```python
from build123d import *

# Parameters (mm, degrees)
ESQUISSE2_R        = 10
ESQUISSE2_R_2      = 1
BOSS_EXTRU_1_DEPTH = 2
BOSS_EXTRU_2_DEPTH = 2


with BuildPart() as part:
    # Esquisse2 → Boss.-Extru.1 (new body)
    with BuildSketch(Plane.XY):
        with Locations((22.149661623, 17.880169066)):
            Circle(ESQUISSE2_R)
        with Locations((16.492807374, 23.537023315)):
            Circle(ESQUISSE2_R_2, mode=Mode.SUBTRACT)
        with Locations((22.149661623, 25.880169066)):
            Circle(ESQUISSE2_R_2, mode=Mode.SUBTRACT)
        with Locations((27.806515873, 23.537023315)):
            Circle(ESQUISSE2_R_2, mode=Mode.SUBTRACT)
        with Locations((30.149661623, 17.880169066)):
            Circle(ESQUISSE2_R_2, mode=Mode.SUBTRACT)
        with Locations((27.806515873, 12.223314816)):
            Circle(ESQUISSE2_R_2, mode=Mode.SUBTRACT)
        with Locations((22.149661623, 9.880169066)):
            Circle(ESQUISSE2_R_2, mode=Mode.SUBTRACT)
        with Locations((16.492807374, 12.223314816)):
            Circle(ESQUISSE2_R_2, mode=Mode.SUBTRACT)
        with Locations((14.149661623, 17.880169066)):
            Circle(ESQUISSE2_R_2, mode=Mode.SUBTRACT)
    extrude(amount=BOSS_EXTRU_1_DEPTH)

    # Esquisse3 → Boss.-Extru.2 (add)
    with BuildSketch(Plane.XY.offset(2)):
        with BuildLine():
            ThreePointArc((26.149661623, 17.880169066), (24.978088748, 20.70859619), (22.149661623, 21.880169066))
            Line((22.149661623, 21.880169066), (22.149661623, 13.880169066))
            ThreePointArc((22.149661623, 13.880169066), (24.978088748, 15.051741941), (26.149661623, 17.880169066))
        make_face()
        with BuildLine():
            Line((22.149661623, 13.880169066), (22.149661623, 21.880169066))
            ThreePointArc((22.149661623, 21.880169066), (18.149661623, 17.880169066), (22.149661623, 13.880169066))
        make_face()
    extrude(amount=BOSS_EXTRU_2_DEPTH)


solid = part.part
```
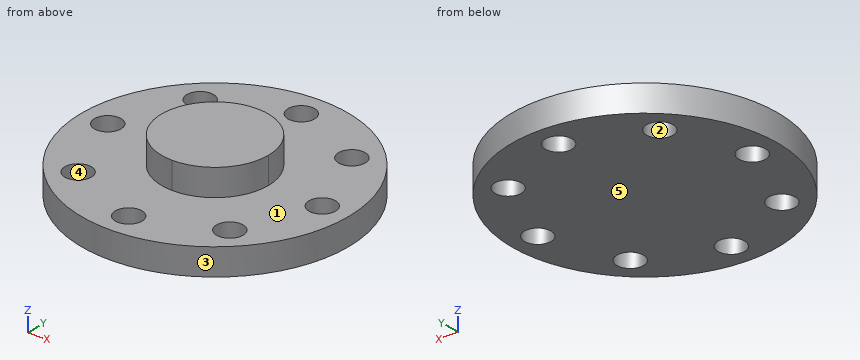
Design review of the part built by this model. Coordinates are the model's own, in mm. Face numbers are marked on the shaded views. A direction names the side the tool comes from. Coordinates: 2 decimals unless noted, no trailing zeros. Write each loop counter-clockwise with the first axis right and the second up, starting at its lowest first coordinate (ties: lowest second). Pieces come first, ordered by that corner, then holes.
1) Mouldability with a two-part tool opening along Y and no side actions: class the marked faces 3, 4 and 5 as +Y half, -Y half, draft (parallel to the pull), parting line (faces both ways), or undercut.
2) Machinability: for the marked faces 1 and 2, which of the approach directions +Z, -Z, +X, -X, +Y, -Y give a long, thin tool a straight path to every point of the face, cutting with its end or side? Answer none if there is none.
3) To check wall thickness, follow L1, parallel to Y at x = 22.5, z = 1.25; L2, parallel to Z at x = 21.25, y = 12.75; L3, parallel to X at y = 22.25, z = 0.2. State the ranges of each line that lie inside material, in increasing order.
4) Add section B-B (x = 30). Write out the cut boundary in (y, z), plus the area to 3 significant figures.
5) Add section D-D (x = 16). Write out the cut boundary in (y, z), plus the area to 3 significant figures.
6) Insertion check: pin 1 (2.5 mm diameter, centred on x = 16.49, y = 23.54, fed in from +Z); pin 2 (1 mm diameter, centred on x = 21, z = 3.5, fed in from +Y). Each pin has a flat end and moves straight along its axis. Give the tip position at first contact, or say it passes through.
7) Add section A-A (y = 25.5). Write out the cut boundary in (x, z).
8) Add section C-C (z = 1). State how many separate pieces and enclosed holes the cut face has, plus the area to 3 significant figures.
Check result:
1. face 3: parting line
1. face 4: undercut
1. face 5: draft
2. face 1: +Z
2. face 2: +Z, -Z
3. L1: y = 7.89 to 8.94, 10.82 to 24.94, 26.82 to 27.87
3. L2: z = 0 to 2
3. L3: x = 13.15 to 31.14
4. outline: (11.69, 0) - (16.89, 0) - (16.89, 2) - (11.69, 2) - close; (18.87, 0) - (24.07, 0) - (24.07, 2) - (18.87, 2) - close
4. area: 20.8 mm2
5. outline: (9.99, 0) - (11.35, 0) - (11.35, 2) - (9.99, 2) - close; (13.09, 0) - (22.67, 0) - (22.67, 2) - (13.09, 2) - close; (24.41, 0) - (25.77, 0) - (25.77, 2) - (24.41, 2) - close
5. area: 24.6 mm2
6. pin 1: stops at z = 2
6. pin 2: stops at y = 21.83
7. outline: (15.67, 0) - (21.22, 0) - (21.22, 2) - (15.67, 2) - close; (23.07, 0) - (28.63, 0) - (28.63, 2) - (23.07, 2) - close
8. separate pieces: 1
8. enclosed holes: 8
8. area: 289 mm2
